The figure shows three views and two pictorial views of one solid part (mm, origin at its lowest corner). Answer the questions. A direction names the side the tool comes from. Coordinates: 2 decimals unless noted, no trailing zeros. Write each loop counter-clockwise with the first axis right and the second up, starting at its lowest first coordinate (ties: lowest second). Pieces come first, ordered by that corner, then holes.
Item 1: Determine the mould class of the marked faces 1, 2, 3 and 4 for opening direction Z: released by +Z, released by -Z, zero draft, split by the parting line, or undercut.
Item 2: Each of these flat-tipped pins is pushed along its axis until it touches: P1, Ø0.8, axis at x = 8.5, z = 8, coming from the +Y side; P2, Ø10, axis at y = 5, z = 15.5, coming from the -X side; P3, Ø4, axis at y = 9, z = 9, coming from the +X side; P4, Ø3.5, axis at y = 9, z = 9, coming from the -X side. Where does it stop, or does it pass through?
Item 3: A tool of negligible diameter and unlimited length cuts with its end or side. For the marked faces 5 and 6, from which of +Z, -Z, +X, -X, +Y, -Y can it reach the whole face along a straight path? Write none if from no direction.
Item 4: Straight lines are drawn through the part: probe 1 along Y at (x, z) = (2.55, 9); probe 2 along X at (y, z) = (2.5, 8.75); probe 3 along Z at (x, y) = (0.75, 7.5). For each, find the intervals that lie inside material, in ascending order.
Item 5: Section C-C (x = 4) is taken. Give the vertices of the cut face in (y, z).
Item 6: Section B-B (x = 5.5) is taken. Give the vertices of the cut face in (y, z).
Item 7: Section A-A (z = 9) is taken. Give the vertices of the cut face in (x, y).
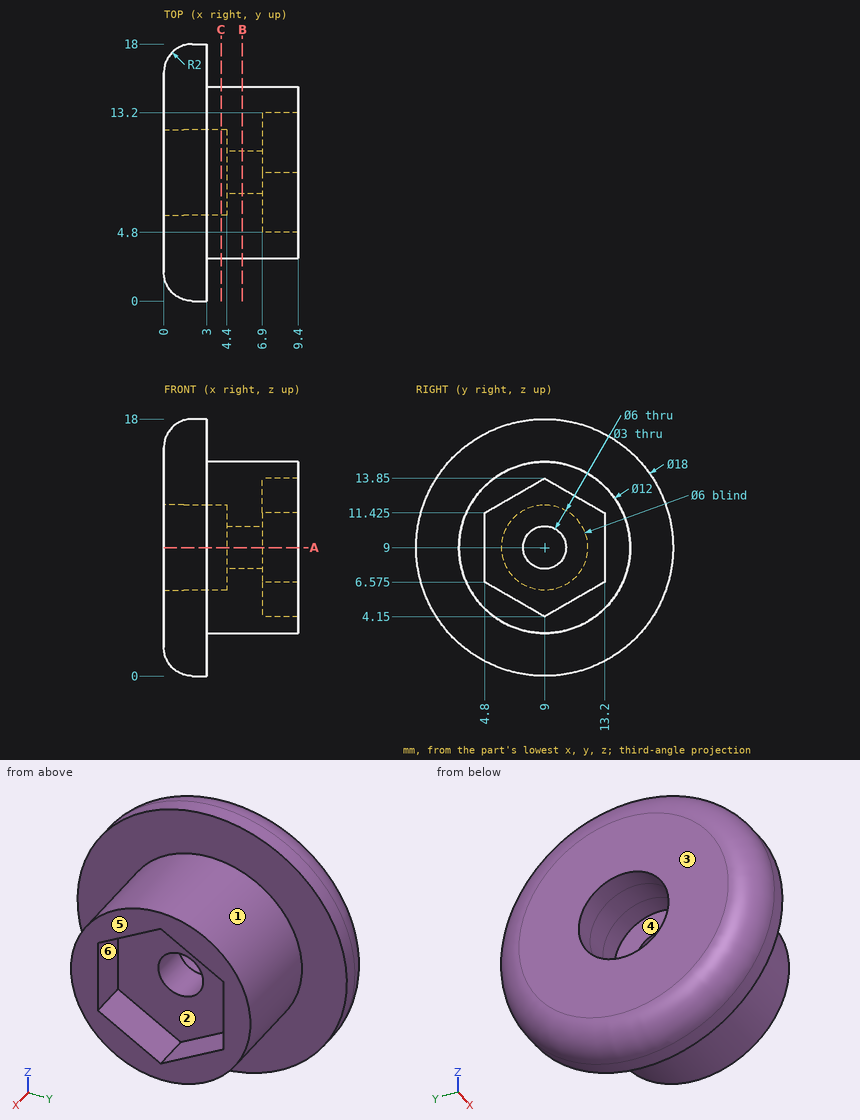
Established:
1. face 1: split by the parting line
1. face 2: undercut
1. face 3: zero draft
1. face 4: undercut
2. P1: stops at y = 14.97
2. P2: stops at x = 0
2. P3: stops at x = 6.9
2. P4: stops at x = 4.4
3. face 5: +Z, -Z, +X, +Y, -Y
3. face 6: +X
4. probe 1: y = 0 to 6, 12 to 18
4. probe 2: x = 0 to 3
4. probe 3: z = 0.57 to 6.4, 11.6 to 17.43
5. outline: circle Ø12 at (9, 9); hole circle Ø6 at (9, 9)
6. outline: circle Ø12 at (9, 9); hole circle Ø3 at (9, 9)
7. outline: (0, 2) arc R2 ccw to (2, 0) - (3, 0) - (3, 3) - (9.4, 3) - (9.4, 4.8) - (6.9, 4.8) - (6.9, 7.5) - (4.4, 7.5) - (4.4, 6) - (0, 6) - close; (0, 12) - (4.4, 12) - (4.4, 10.5) - (6.9, 10.5) - (6.9, 13.2) - (9.4, 13.2) - (9.4, 15) - (3, 15) - (3, 18) - (2, 18) arc R2 ccw to (0, 16) - close
